Read the model definition and answer for the solid it produces. Units are mm, in the model's axes. A direction names the side the tool comes from. Round coordinates to 2 decimals unless told otherwise and drop trailing zeros. Order: outer loops, then holes, each group sorted by start corner. A loop starts at its lowest first (then second) coordinate and runs counter-clockwise, first axis right, second up. Notation, with made-up numbers: M -2,27.25 L 25,27.25 A14 cw 25,45.25 Z; hole C 66.5,39 d1. An arc over 180 degrees is marked long. Use one line per item in the form item = value. Start each with the question number.
from build123d import *

# Parameters (mm, degrees)
BOSS_EXTRUDE1_DEPTH                = 12.7
F_5_16_18_TAPPED_HOLE1_D           = 6.5278
F_5_16_18_TAPPED_HOLE1_DEPTH       = 20.1168
F_5_16_18_TAPPED_HOLE1_CSINK_D     = 7.9375
F_5_16_18_TAPPED_HOLE1_CSINK_ANGLE = 90
F_5_16_18_TAPPED_HOLE1_TIP         = 1.961148974
SKETCH8_OUTSIDE_W                  = 77.69
SKETCH8_OUTSIDE_H                  = 153.891
CUT_EXTRUDE1_DEPTH                 = 229.6
FILLET1_R                          = 2.38125


with BuildPart() as part:
    # Sketch1 w/mock PCB → Boss-Extrude1 (new body, symmetric)
    with BuildSketch(Plane.XY):
        Polygon((-19.05, 48.1965), (-228.6, -28.0035), (-228.6, -44.5135), (-195.422068321, -53.4035), (-33.177931679, -53.4035), (0, -44.5135), (0, 48.1965), align=None)
        with BuildLine():
            Line((-20.32, 12.51406647), (-20.32, -23.5585))
            ThreePointArc((-20.32, -23.5585), (-23.109807909, -30.293692091), (-29.845, -33.0835))
            Line((-29.845, -33.0835), (-129.044557791, -33.0835))
            ThreePointArc((-129.044557791, -33.0835), (-138.425095375, -25.211115999), (-132.299660467, -14.606967641))
            Line((-132.299660467, -14.606967641), (-33.100102676, 21.465598828))
            ThreePointArc((-33.100102676, 21.465598828), (-24.380534243, 20.315684186), (-20.32, 12.51406647))
        make_face(mode=Mode.SUBTRACT)
    extrude(amount=BOSS_EXTRUDE1_DEPTH, both=True)

    # 5/16-18 Tapped Hole1
    with Locations(Plane(origin=(0, 31.393459191, 0.765177918), x_dir=(0, 0, 1), z_dir=(1, 0, 0))):
        with Locations((-0.765177918, 69.493459191), (-0.765177918, 25.856259191), (-0.765177918, -6.706540809)):
            CounterSinkHole(F_5_16_18_TAPPED_HOLE1_D / 2, F_5_16_18_TAPPED_HOLE1_CSINK_D / 2, depth=F_5_16_18_TAPPED_HOLE1_DEPTH, counter_sink_angle=F_5_16_18_TAPPED_HOLE1_CSINK_ANGLE)
            with Locations((0, 0, -(F_5_16_18_TAPPED_HOLE1_DEPTH + F_5_16_18_TAPPED_HOLE1_TIP / 2))):  # 118° drill point
                Cone(0, F_5_16_18_TAPPED_HOLE1_D / 2, F_5_16_18_TAPPED_HOLE1_TIP, mode=Mode.SUBTRACT)

    # Sketch8 outside → Cut-Extrude1 (cut, through all)
    with BuildSketch(Plane(origin=(0, 0, 0), x_dir=(0, 0, -1), z_dir=(1, 0, 0))):
        with Locations((0, -2.6035)):
            Rectangle(SKETCH8_OUTSIDE_W, SKETCH8_OUTSIDE_H)
        with BuildLine():
            Line((12.7, 48.1965), (12.7, -51.725281086))
            ThreePointArc((12.7, -51.725281086), (0, -51.816), (-12.7, -51.725281086))
            Line((-12.7, -51.725281086), (-12.7, 48.1965))
            Line((-12.7, 48.1965), (12.7, 48.1965))
        make_face(mode=Mode.SUBTRACT)
    extrude(amount=-CUT_EXTRUDE1_DEPTH, mode=Mode.SUBTRACT)

    # Fillet1
    fillet1_edges = [part.edges().sort_by_distance(p)[0] for p in [
        (-114.3, -51.725281086, -12.7),
        (-114.3, -51.725281086, 12.7),
    ]]
    fillet(fillet1_edges, radius=FILLET1_R)


solid = part.part
Item 1: Section A-A (x = -86) is taken. Write down the section's boundary in (y, z), and give its area (3 significant figures).
Item 2: Find the intervals of material crossed by L1, parallel to Z at x = -16, y = 38; L2, parallel to Y at x = -11.75, z = 0; L3, parallel to Y at x = -14.5, z = 0, in increasing order. Write a range as [from, to].
Item 3: Given P1, Ø1, axis at x = -197, z = 6, coming from the +Y side; P2, Ø12.5, axis at x = -89.5, z = 1.5, coming from the +Y side; P3, Ø2, axis at x = -47, z = -7, coming from the -Y side, each flat-ended and moving along its own axis, determine where each tip first touches the part or whether it passes through.
Item 4: Section C-C (y = 31) is taken. Write down the section's boundary in (x, z), and give its area (3 significant figures).
Item 5: For a pull along X with two mould halves and no side action, classify faces 1 (the flat face through (-215.164, -48.114, 0.178)), 2 (the flat face through (-79, -33.084, 0)), 3 (the cylindrical face through (-10.547, 41.286, 0.708)) as pulls with the +X half, pulls with the -X half, needs draft (parallel to the pull), parting line crosses it, or undercut.
Item 6: Section D-D (x = -169) is taken. Write down the section's boundary in (y, z).
Item 7: A tool of negligible diameter and unlimited length cuts with its end or side. For faces 4 (the cylindrical face through (-10.547, 8.723, 0.708)), 5 (the cylindrical face through (-138.39, -25.39, 0.18)), 6 (the flat face through (-228.6, -36, 0)), from which of +Z, -Z, +X, -X, +Y, -Y can it reach the whole face along a straight path? Write none if from no direction.
Item 8: Section B-B (x = -194.5) is taken. Write down the section's boundary in (y, z), and give its area (3 significant figures).
The answers:
q1.outline = M -51.76,-10.35 A2.38 ccw -49.37,-12.7 L -33.08,-12.7 L -33.08,12.7 L -49.37,12.7 A2.38 ccw -51.76,10.35 A889 ccw Z; M 2.23,-12.7 L 23.85,-12.7 L 23.85,12.7 L 2.23,12.7 Z
q1.area = 1,020 mm²
q2.L1 = [-12.7, -3.26], [3.26, 12.7]
q2.L2 = [-47.66, -41.36], [-34.84, 2.27], [8.8, 34.84], [41.36, 48.2]
q2.L3 = [-48.4, -41.36], [-34.84, 2.27], [8.8, 34.84], [41.36, 48.2]
q3.P1 = -16.33
q3.P2 = 24.85
q3.P3 = -51.8
q4.outline = M -66.34,-12.7 L 0,-12.7 L 0,12.7 L -66.34,12.7 Z
q4.area = 1,690 mm²
q5.face_1 = pulls with the -X half
q5.face_2 = undercut
q5.face_3 = needs draft
q6.outline = M -51.76,-10.35 A2.38 ccw -49.37,-12.7 L -6.33,-12.7 L -6.33,12.7 L -49.37,12.7 A2.38 ccw -51.76,10.35 A889 ccw Z
q7.face_4 = +X
q7.face_5 = +Z, -Z
q7.face_6 = +Z, -Z, -X, +Y, -Y
q8.outline = M -51.76,-10.35 A2.38 ccw -49.37,-12.7 L -15.6,-12.7 L -15.6,12.7 L -49.37,12.7 A2.38 ccw -51.76,10.35 A889 ccw Z
q8.area = 917 mm²
